from build123d import *

# Parameters (mm, degrees)
SKETCH1_W           = 400
SKETCH1_H           = 400
BOSS_EXTRUDE1_DEPTH = 50
SKETCH3_W           = 200
SKETCH3_H           = 200
BOSS_EXTRUDE2_DEPTH = 50
SKETCH4_W           = 95
SKETCH4_H           = 95
CUT_EXTRUDE1_DEPTH  = 45
SKETCH6_R           = 10
BOSS_EXTRUDE4_DEPTH = 10
LPATTERN3_COUNT     = 5
LPATTERN3_PITCH     = 25
SKETCH7_W           = 50
SKETCH7_H           = 50
BOSS_EXTRUDE5_DEPTH = 25
SKETCH8_R           = 15
BOSS_EXTRUDE6_DEPTH = 15
SKETCH10_W          = 50
SKETCH10_H          = 50
BOSS_EXTRUDE7_DEPTH = 50
SKETCH12_W          = 30
SKETCH12_H          = 30
CUT_EXTRUDE2_DEPTH  = 45
SKETCH13_W          = 50
SKETCH13_H          = 50
BOSS_EXTRUDE8_DEPTH = 50


with BuildPart() as part:
    # Sketch1 → Boss-Extrude1 (new body)
    with BuildSketch(Plane(origin=(0, 0, 0), x_dir=(1, 0, 0), z_dir=(0, 1, 0))):
        Rectangle(SKETCH1_W, SKETCH1_H)
    extrude(amount=BOSS_EXTRUDE1_DEPTH)

    # Sketch3 → Boss-Extrude2 (add)
    with BuildSketch(Plane(origin=(0, 50, 0), x_dir=(1, 0, 0), z_dir=(0, 1, 0))):
        Rectangle(SKETCH3_W, SKETCH3_H)
    extrude(amount=BOSS_EXTRUDE2_DEPTH)

    # Sketch4 → Cut-Extrude1 (cut)
    with BuildSketch(Plane(origin=(0, 100, 0), x_dir=(1, 0, 0), z_dir=(0, 1, 0))):
        with Locations((-50, -50)):
            Rectangle(SKETCH4_W, SKETCH4_H)
        with Locations((50, -50)):
            Rectangle(SKETCH4_W, SKETCH4_H)
        with Locations((-50, 50)):
            Rectangle(SKETCH4_W, SKETCH4_H)
        with Locations((50, 50)):
            Rectangle(SKETCH4_W, SKETCH4_H)
    extrude(amount=-CUT_EXTRUDE1_DEPTH, mode=Mode.SUBTRACT)

    # Sketch6 → Boss-Extrude4 (add)
    with BuildSketch(Plane(origin=(0, 50, 0), x_dir=(1, 0, 0), z_dir=(0, 1, 0))):
        with Locations(Location((180, -180, 0), (0, 0, 270))):
            Circle(SKETCH6_R)
    boss_extrude4 = extrude(amount=BOSS_EXTRUDE4_DEPTH)

    # LPattern3: Boss-Extrude4 ×5
    with Locations(*[(0, 0, -i * LPATTERN3_PITCH) for i in range(1, LPATTERN3_COUNT)]):
        add(boss_extrude4)

    # Sketch7 → Boss-Extrude5 (add)
    with BuildSketch(Plane(origin=(0, 50, 0), x_dir=(1, 0, 0), z_dir=(0, 1, 0))):
        with Locations((133.117890176, -156.630485574)):
            Rectangle(SKETCH7_W, SKETCH7_H)
    extrude(amount=BOSS_EXTRUDE5_DEPTH)

    # Sketch8 → Boss-Extrude6 (add)
    with BuildSketch(Plane(origin=(0, 75, 0), x_dir=(1, 0, 0), z_dir=(0, 1, 0))):
        with Locations(Location((133.117890176, -156.630485574, 0), (0, 0, 270))):
            Circle(SKETCH8_R)
    extrude(amount=BOSS_EXTRUDE6_DEPTH)

    # Sketch10 → Boss-Extrude7 (add)
    with BuildSketch(Plane(origin=(0, 50, 0), x_dir=(1, 0, 0), z_dir=(0, 1, 0))):
        with Locations((-165.022837079, -166.245313822)):
            Rectangle(SKETCH10_W, SKETCH10_H)
    extrude(amount=BOSS_EXTRUDE7_DEPTH)

    # Sketch12 → Cut-Extrude2 (cut)
    with BuildSketch(Plane(origin=(0, 100, 0), x_dir=(1, 0, 0), z_dir=(0, 1, 0))):
        with Locations((-164.276921981, -166.025383847)):
            Rectangle(SKETCH12_W, SKETCH12_H)
    extrude(amount=-CUT_EXTRUDE2_DEPTH, mode=Mode.SUBTRACT)

    # Sketch13 → Boss-Extrude8 (add)
    with BuildSketch(Plane(origin=(0, 50, 0), x_dir=(1, 0, 0), z_dir=(0, 1, 0))):
        with Locations((-90.022837079, -166.245313822)):
            Rectangle(SKETCH13_W, SKETCH13_H)
    extrude(amount=BOSS_EXTRUDE8_DEPTH)


solid = part.part
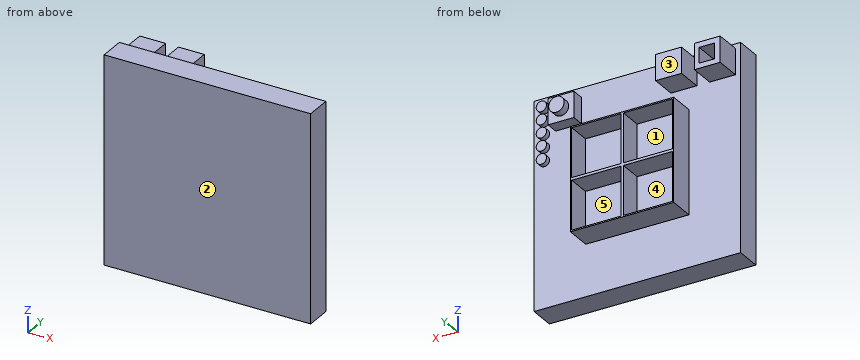
Read the model definition and answer for the solid it produces. Units are mm, in the model's axes. Face numbers are marked on the shaded views. A direction names the side the tool comes from. Round coordinates to 2 decimals unless told otherwise and drop trailing zeros. Loops run counter-clockwise (first coordinate to the right, second up) from the corner with the lowest first, then second, coordinate; pieces in that order, holes last.
Q1. Section C-C on x = 85 is taken. Write down the section's boundary in (y, z).
Q2. Section A-A on y = 68 is taken. Give the number of separate pieces and of enclosed holes in the cut face, and give its area (3 significant figures).
Q3. Determine the mould class of the marked faces 3, 4 and 5 for opening direction X: released by +X, released by -X, zero draft, split by the parting line, or undercut.
Q4. Section B-B on z = 105 is taken. Write down the section's boundary in (x, y).
Q5. Which of the six approach directions +Z, -Z, +X, -X, +Y, -Y give full straight-line access (tool end or side, diameter ignored) to the marked faces 1 and 2?
Q6. Consider probe 1 along Z at (x, y) = (21, 82.5); probe 2 along Y at (x, z) = (-136.5, -65). Determine where each line is inside the solid, lowest interval first.
Q7. Section D-D on x = 180 is taken. Write down the section's boundary in (y, z), and give its area (3 significant figures).
Q8. Each of these flat-tipped pins is pushed along its axis until it touches: pin 1 (22.5 mm diameter, centred on y = 70, z = -63, fed in from -X); pin 2 (22 mm diameter, centred on x = 180.5, z = 109, fed in from +Y); pin 3 (15 mm diameter, centred on x = -177.5, y = 72, fed in from -Z). Where does it stop, or does it pass through?
Output:
1. outline: (0, -200) - (50, -200) - (50, -100) - (100, -100) - (100, -97.5) - (55, -97.5) - (55, -2.5) - (100, -2.5) - (100, 2.5) - (55, 2.5) - (55, 97.5) - (100, 97.5) - (100, 100) - (50, 100) - (50, 200) - (0, 200) - close
2. separate pieces: 4
2. enclosed holes: 5
2. area: 10,500 mm2
3. face 3: zero draft
3. face 4: undercut
3. face 5: undercut
4. outline: (-200, 0) - (200, 0) - (200, 50) - (190, 50) - (190, 60) - (170, 60) - (170, 50) - (-200, 50) - close
5. face 1: +Y
5. face 2: +Z, -Z, +X, -X, -Y
6. probe 1: z = -100 to -97.5, -2.5 to 2.5, 97.5 to 100
6. probe 2: y = 0 to 50
7. outline: (0, -200) - (50, -200) - (50, 70) - (60, 70) - (60, 90) - (50, 90) - (50, 95) - (60, 95) - (60, 115) - (50, 115) - (50, 120) - (60, 120) - (60, 140) - (50, 140) - (50, 145) - (60, 145) - (60, 165) - (50, 165) - (50, 170) - (60, 170) - (60, 190) - (50, 190) - (50, 200) - (0, 200) - close
7. area: 21,000 mm2
8. pin 1: stops at x = -100
8. pin 2: stops at y = 60
8. pin 3: stops at z = 141.25
